Autodesk Inventor part; units mm, degrees
ref_plane "YZ Plane" through (0, 0, 0) normal (1, 0, 0) x (0, 1, 0)
ref_plane "XZ Plane" through (0, 0, 0) normal (0, 1, 0) x (-1, 0, 0)
ref_plane "XY Plane" through (0, 0, 0) normal (0, 0, 1) x (1, 0, 0)
sketch "Sketch1" plane through (0, 0, 0) normal (1, 0, 0) x (0, 1, 0)
  line L0 (-9.525, 4.7625) -> (9.525, 4.7625) construction
  line L1 (9.525, 4.7625) -> (9.525, -4.7625) construction
  line L2 (9.525, -4.7625) -> (-9.525, -4.7625) construction
  line L3 (-9.525, -4.7625) -> (-9.525, 4.7625) construction
  line L4 (-9.525, 4.7625) -> (9.525, -4.7625) construction
  line L5 (9.525, 4.7625) -> (-9.525, -4.7625) construction
  line L6 (-9.779, 4.7625) -> (9.779, 4.7625)
  line L7 (9.779, 4.7625) -> (9.779, -4.7625)
  line L8 (9.779, -4.7625) -> (-9.779, -4.7625) construction
  line L9 (-9.779, -4.7625) -> (-9.779, 4.7625)
  line L10 (-9.779, 4.7625) -> (9.779, -4.7625) construction
  line L11 (9.779, 4.7625) -> (-9.779, -4.7625) construction
  line L12 (-14.2875, 11.1125) -> (14.2875, 11.1125)
  line L13 (14.2875, 11.1125) -> (14.2875, -4.7625)
  line L14 (14.2875, -4.7625) -> (-14.2875, -4.7625)
  line L15 (-14.2875, -4.7625) -> (-14.2875, 11.1125)
  line L16 (-14.2875, 11.1125) -> (14.2875, -4.7625) construction
  line L17 (14.2875, 11.1125) -> (-14.2875, -4.7625) construction
  line L18 (0, 4.7625) -> (0, 0) construction
  line L19 (-14.2875, 11.1125) -> (-11.1125, 11.1125)
  line L20 (-11.1125, 11.1125) -> (-11.1125, 33.3375)
  line L21 (-11.1125, 33.3375) -> (-14.2875, 33.3375)
  line L22 (-14.2875, 33.3375) -> (-14.2875, 11.1125)
  line L23 (-14.2875, 33.3375) -> (-11.1125, 33.3375)
  line L24 (-11.1125, 33.3375) -> (-11.1125, 36.5125) construction
  line L25 (-11.1125, 36.5125) -> (-14.2875, 36.5125)
  line L26 (-14.2875, 36.5125) -> (-14.2875, 33.3375)
  circle A0 centre (-11.1125, 34.925) radius 1.5875
  circle A1 centre (8.6565, 3.64) radius 1.5875
  line L27 (8.6565, 3.64) -> (9.779, 4.7625) construction
  circle A2 centre (-8.6565, 3.64) radius 1.5875
  line L28 (-11.1125, 33.3375) -> (-9.525, 33.3375)
  line L29 (-9.525, 33.3375) -> (-9.525, 34.925)
  line L30 (-9.525, 34.925) -> (-11.1125, 34.925) construction
  line L31 (-11.1125, 34.925) -> (-11.1125, 33.3375)
  point P0 (0, 3.175)
  point P1 (-9.779, 2.5174)
  point P2 (-7.5339, 4.7625)
  point P3 (7.5339, 4.7625)
  point P4 (9.779, 2.5174)
  dimension "d11" = 3.175
  dimension "d0" = 19.05
  dimension "d1" = 9.525
  dimension "d2" = 19.558
  dimension "d3" = 6.35
  dimension "d4" = 28.575
  dimension "d5" = 3.175
  dimension "d6" = 22.225
  dimension "d7" = 3.175
  dimension "d8" = 3.175
extrude "Extrusion1" add sketch "Sketch1" along normal blind 25.4 contours A2 L9 L14 L15 L12 L13 L7 A1 L6 | L22 L21 L20 L12 | L26 L25 A0 L21 | A0 | A0 L29 L28
chamfer "Chamfer1" distance 0.3969 angle 45 3 edges at (12.7, -9.779, -4.7625) (12.7, 9.779, -4.7625) (12.7, -9.525, 33.3375)
fillet "Fillet1" radius 2.3813 2 edges at (12.7, 14.2875, -4.7625) (12.7, -14.2875, -4.7625)
fillet "Fillet2" radius 2.3813 1 edges at (12.7, 14.2875, 11.1125)
sketch "Sketch2" plane through (0, -11.1125, 11.1125) normal (0, 0, 1) x (1, 0, 0)
  line L0 (0, 23.0188) -> (0, 0)
  line L1 (0, 12.7) -> (25.4, 12.7) construction
  line L2 (25.4, 3.5786) -> (25.4, 18.6464)
  line L3 (25.4, 25.4) -> (0, 25.4)
  point P0 (0, 11.1125)
  point P1 (6.35, 12.7)
  point P2 (19.05, 12.7)
  dimension "d17" = 12.7
  dimension "d18" = 6.35
  dimension "d21" = 12.7
hole "Hole1" at (6.35, 1.5875, 11.1125) at (19.05, 1.5875, 11.1125) direction (0, 0, -1) diameter 3.81 end through all countersink diameter 7.62 countersink angle 82
properties part number "Door Bracket"
Here's how the part is built. I have some questions about the finished solid (model axes, mm). A direction names the side the tool comes from. Coordinates: 2 decimals unless noted, no trailing zeros. Order: outer loops, then holes, each group sorted by start corner. A loop starts at its lowest first (then second) coordinate and runs counter-clockwise, first axis right, second up. Notation, with made-up numbers: (70, -12) - (118, -12) arc R27 ccw to (118, 19) - close; hole circle Ø11 at (2, -40). An arc over 180 degrees is marked (long way). Use CSV: the item, a comma, the result in double quotes. Start each with the question number.
1. Suppose I cut it at D-D on z = 25. List the corners of the cut face in (x, y) for me.
2. For faces 3 (the face through (13, -11.112, 22)), 4 (the face through (13, -9.525, 34)), 5 (the face through (12.878, -13.608, -4.046)), 6 (the face through (13, -9.779, -1)), which set-ups out of +Z, -Z, +X, -X, +Y, -Y let a thin tool reach every point of the face, with its end or its side?
3. Suppose I cut it at B-B on x = 19.05. List the corners of the cut face in (y, z) for me (1 decimal), then the cut area to 3 significant figures.
4. If we mould it in two halves opening along X, with no side actions, what happens to faces 1 (the face through (13, 0, 4.762)), 2 (the face through (17.818, 3.194, 9.058))? For each: +X half, -X half, draft (parallel to the pull), parting line (faces both ways), or undercut.
5. Suppose I cut it at A-A on z = 3.64. List the corners of the cut face in (x, y) for me, then the cut area to 3 significant figures.
6. Please list where these lines run through material, in increasing order: line 1 (Y direction, x = 17, z = 2.5); line 2 (Y direction, x = 19.05, z = 6.6); line 3 (Y direction, x = 18.5, z = 27.5). Write a range as from..to.
7. I'm going to push flat-ended pins straight in: pin 1 (8 mm diameter, centred on x = 3.5, z = 26, fed in from +Y); pin 2 (8 mm diameter, centred on x = 21, y = -3, fed in from -Z); pin 3 (11.5 mm diameter, centred on x = 18.5, y = -2, fed in from +Z). Where does each tip first touch, or does it pass through?
8. Suppose I cut it at C-C on x = 12.5. List the corners of the cut face in (y, z) for me (1 decimal).
Output:
1,outline,"(0, -14.29) - (25.4, -14.29) - (25.4, -11.11) - (0, -11.11) - close"
2,face 3,"+X, -X, +Y"
2,face 4,"+Z, +X, -X, +Y"
2,face 5,"-Z, +X, -X, -Y"
2,face 6,"-Z, +X, -X"
3,outline,"(-14.3, -2.4) arc R2.4 ccw to (-11.9, -4.8) - (-10.2, -4.8) - (-9.8, -4.4) - (-9.8, 2.5) arc R1.6 cw to (-7.5, 4.8) - (-0.3, 4.8) - (-0.3, 8.9) - (-2.2, 11.1) - (-11.1, 11.1) - (-11.1, 33.3) - (-9.9, 33.3) - (-9.5, 33.7) - (-9.5, 34.9) arc R1.6 ccw to (-11.1, 36.5) - (-14.3, 36.5) - close; (3.5, 4.8) - (7.5, 4.8) arc R1.6 cw to (9.8, 2.5) - (9.8, -4.4) - (10.2, -4.8) - (11.9, -4.8) arc R2.4 ccw to (14.3, -2.4) - (14.3, 8.7) arc R2.4 ccw to (11.9, 11.1) - (5.4, 11.1) - (3.5, 8.9) - close"
3,area,"317 mm2"
4,face 1,"draft"
4,face 2,"undercut"
5,outline,"(0, -14.29) - (25.4, -14.29) - (25.4, -10.24) - (0, -10.24) - close; (0, 10.24) - (25.4, 10.24) - (25.4, 14.29) - (0, 14.29) - close"
5,area,"205 mm2"
6,line 1,"y = -14.29..-9.78, 9.78..14.29"
6,line 2,"y = -14.29..-0.32, 3.49..14.29"
6,line 3,"y = -14.29..-11.11"
7,pin 1,"stops at y = -11.11"
7,pin 2,"stops at z = 4.76"
7,pin 3,"stops at z = 11.11"
8,outline,"(-14.3, -2.4) arc R2.4 ccw to (-11.9, -4.8) - (-10.2, -4.8) - (-9.8, -4.4) - (-9.8, 2.5) arc R1.6 cw to (-7.5, 4.8) - (7.5, 4.8) arc R1.6 cw to (9.8, 2.5) - (9.8, -4.4) - (10.2, -4.8) - (11.9, -4.8) arc R2.4 ccw to (14.3, -2.4) - (14.3, 8.7) arc R2.4 ccw to (11.9, 11.1) - (-11.1, 11.1) - (-11.1, 33.3) - (-9.9, 33.3) - (-9.5, 33.7) - (-9.5, 34.9) arc R1.6 ccw to (-11.1, 36.5) - (-14.3, 36.5) - close"
